Read the model definition and answer for the solid it produces. Units are mm, in the model's axes. Face numbers are marked on the shaded views. A direction names the side the tool comes from. Give positions to 0.01 mm unless a question says otherwise; leave off trailing zeros. Loops run counter-clockwise (first coordinate to the right, second up) from the corner with the lowest first, then second, coordinate; pieces in that order, holes last. Notation, with made-up numbers: (1.5, -1.75) - (25.5, -1.75) arc R16 cw to (25.5, 22.25) - close; hole circle Ø5 at (-32, 64.25). An arc over 180 degrees is marked (long way). Write item = value, one per line. Start each with the question number.
from build123d import *

# Parameters (mm, degrees)
SKETCH_1_R           = 20.68
SKETCH_1_R_2         = 9.68
EXTRUDE_1_DEPTH      = 116.68
SKETCH_11_W          = 27
SKETCH_11_H          = 150
CUT_EXTRUDE_3_DEPTH  = 40
SKETCH_13_W          = 10
SKETCH_13_H          = 128.345013401
CUT_EXTRUDE_7_DEPTH  = 126.614916312
SKETCH_15_W          = 8
SKETCH_15_H          = 68.68
CUT_EXTRUDE_9_DEPTH  = 48
SKETCH_16_W          = 15.549431524
SKETCH_16_H          = 20
SKETCH_16_W_2        = 15.459431524
EXTRUDE_4_DEPTH      = 19.2
SKETCH_17_W          = 19.20851187
SKETCH_17_H          = 14.03
CUT_EXTRUDE_10_DEPTH = 20.2
SKETCH_18_R          = 9.59
CUT_EXTRUDE_11_DEPTH = 121.289430957
SKETCH_21_R          = 2.985
CUT_EXTRUDE_12_DEPTH = 55.2
EXTRUDE_START        = 55.2
SKETCH_24_R          = 20.59
SKETCH_24_R_2        = 9.59
EXTRUDE_2_DEPTH      = 55.2
CUT_EXTRUDE_13_DEPTH = 55.2
SKETCH_26_W          = 10.00851187
SKETCH_26_H          = 41.68
CUT_EXTRUDE_15_DEPTH = 55.2
SKETCH_27_W          = 10
SKETCH_27_H          = 40
CUT_EXTRUDE_16_DEPTH = 55.2
SKETCH_28_W          = 44.880694938
SKETCH_28_H          = 9.608044066
CUT_EXTRUDE_17_DEPTH = 12.2
SKETCH_35_W          = 13.53
SKETCH_35_H          = 20
EXTRUDE_10_DEPTH     = 15
EXTRUDE_11_DEPTH     = 15
SKETCH_37_W          = 9
SKETCH_37_H          = 20
EXTRUDE_12_DEPTH     = 20
SKETCH_38_W          = 9
SKETCH_38_H          = 20
EXTRUDE_13_DEPTH     = 20
SKETCH_42_R          = 2.985
CUT_EXTRUDE_21_DEPTH = 20
CUT_EXTRUDE_23_DEPTH = 138.235841092
SKETCH_45_W          = 3
SKETCH_45_H          = 20
EXTRUDE_14_DEPTH     = 30
SKETCH_46_W          = 3
SKETCH_46_H          = 20
EXTRUDE_15_DEPTH     = 30
SKETCH_47_W          = 33.078221107
SKETCH_47_H          = 20
EXTRUDE_16_DEPTH     = 50
SKETCH_48_W          = 30
SKETCH_48_H          = 20
EXTRUDE_17_DEPTH     = 50
SKETCH_50_W          = 50
SKETCH_50_H          = 20
EXTRUDE_18_DEPTH     = 1
SKETCH_51_W          = 50
SKETCH_51_H          = 20
EXTRUDE_19_DEPTH     = 1
SKETCH_52_W          = 53
SKETCH_52_H          = 14
CUT_EXTRUDE_24_DEPTH = 151.972575738
SKETCH_53_W          = 53
SKETCH_53_H          = 14
CUT_EXTRUDE_25_DEPTH = 151.942387436
SKETCH_54_W          = 40
SKETCH_54_H          = 73.27
CUT_EXTRUDE_26_DEPTH = 147.866192927
SKETCH_56_W          = 13.00851187
SKETCH_56_H          = 20
EXTRUDE_21_DEPTH     = 3.08
SKETCH_58_W          = 44.672014854
SKETCH_58_H          = 95.939897673
CUT_EXTRUDE_28_DEPTH = 149.701311438
SKETCH_59_R          = 9.7
CUT_EXTRUDE_29_DEPTH = 60.553551814
SKETCH_60_W          = 6.504255935
SKETCH_60_H          = 76.35
CUT_EXTRUDE_30_DEPTH = 60.553551814
CUT_EXTRUDE_32_DEPTH = 20
SKETCH_64_W          = 16.20851187
SKETCH_64_H          = 0.09
EXTRUDE_22_DEPTH     = 20
SKETCH_65_W          = 3.495744065
SKETCH_65_H          = 3.26
CUT_EXTRUDE_33_DEPTH = 58.582567932
SKETCH_66_W          = 3.495744065
SKETCH_66_H          = 1.776778893
SKETCH_66_W_2        = 3.503635083
SKETCH_66_H_2        = 1.775
EXTRUDE_23_DEPTH     = 20.2
SKETCH_68_W          = 6.504255935
SKETCH_68_H          = 3.66
CUT_EXTRUDE_34_DEPTH = 20
SKETCH_69_R          = 2.985
CUT_EXTRUDE_35_DEPTH = 124.351086443
SKETCH_70_R          = 2.985
CUT_EXTRUDE_36_DEPTH = 131.530092773


with BuildPart() as part:
    # 草圖1 → 伸長-薄件1 (new body)
    with BuildSketch(Plane(origin=(0, 0, 0), x_dir=(1, 0, 0), z_dir=(0, 1, 0))):
        Circle(SKETCH_1_R)
        Circle(SKETCH_1_R_2, mode=Mode.SUBTRACT)
    extrude(amount=EXTRUDE_1_DEPTH)

    # 草圖11 → 除料-伸長3 (cut)
    with BuildSketch(Plane(origin=(0, 116.68, 0), x_dir=(1, 0, 0), z_dir=(0, 1, 0))):
        with Locations((21.70851187, -44.235815192)):
            Rectangle(SKETCH_11_W, SKETCH_11_H)
    extrude(amount=-CUT_EXTRUDE_3_DEPTH, mode=Mode.SUBTRACT)

    # 草圖13 → 除料-伸長7 (cut, through all)
    with BuildSketch(Plane.XY.offset(21)):
        with Locations((-16, 58.612182466)):
            Rectangle(SKETCH_13_W, SKETCH_13_H)
    extrude(amount=-CUT_EXTRUDE_7_DEPTH, mode=Mode.SUBTRACT)

    # 草圖15 → 除料-伸長9 (cut)
    with BuildSketch(Plane.XY.offset(21)):
        with Locations((-1.395744065, 52.34)):
            Rectangle(SKETCH_15_W, SKETCH_15_H)
    extrude(amount=-CUT_EXTRUDE_9_DEPTH, mode=Mode.SUBTRACT)

    # 草圖16 → 填料-伸長4 (add)
    with BuildSketch(Plane(origin=(8.20851187, 0, 0), x_dir=(0, 0, -1), z_dir=(1, 0, 0))):
        with Locations((12.905284238, 106.68)):
            Rectangle(SKETCH_16_W, SKETCH_16_H)
        with Locations((-12.860284238, 106.68)):
            Rectangle(SKETCH_16_W_2, SKETCH_16_H)
    extrude(amount=-EXTRUDE_4_DEPTH)

    # 草圖17 → 除料-伸長10 (cut)
    with BuildSketch(Plane(origin=(0, 116.68, 0), x_dir=(1, 0, 0), z_dir=(0, 1, 0))):
        with Locations((-1.395744065, -0.045)):
            Rectangle(SKETCH_17_W, SKETCH_17_H)
    extrude(amount=-CUT_EXTRUDE_10_DEPTH, mode=Mode.SUBTRACT)

    # 草圖18 → 除料-伸長11 (cut, through all)
    with BuildSketch(Plane.XZ):
        with Locations(Location((0, 0, 0), (0, 0, 90))):
            Circle(SKETCH_18_R)
    extrude(amount=-CUT_EXTRUDE_11_DEPTH, mode=Mode.SUBTRACT)

    # 草圖21 → 除料-伸長12 (cut)
    with BuildSketch(Plane(origin=(0, 0, -20.68), x_dir=(-1, 0, 0), z_dir=(0, 0, -1))):
        with Locations((1.39148813, 108.73)):
            Circle(SKETCH_21_R)
    extrude(amount=-CUT_EXTRUDE_12_DEPTH, mode=Mode.SUBTRACT)

    # 草圖24 → 伸長-薄件2 (add)
    with BuildSketch(Plane.XZ.offset(EXTRUDE_START)):
        Circle(SKETCH_24_R)
        Circle(SKETCH_24_R_2, mode=Mode.SUBTRACT)
    extrude(amount=-EXTRUDE_2_DEPTH)

    # 草圖25 → 除料-伸長13 (cut)
    with BuildSketch(Plane.XY.offset(21)):
        Polygon((-1.39148813, -11.785), (22.612379708, -11.785), (22.612379708, -63.873337429), (-22.749525245, -63.873337429), (-22.749525245, -11.785), align=None)
    extrude(amount=-CUT_EXTRUDE_13_DEPTH, mode=Mode.SUBTRACT)

    # 草圖26 → 除料-伸長15 (cut)
    with BuildSketch(Plane(origin=(0, 0, 0), x_dir=(1, 0, 0), z_dir=(0, 1, 0))):
        with Locations((-15.995744065, -0.16)):
            Rectangle(SKETCH_26_W, SKETCH_26_H)
    extrude(amount=-CUT_EXTRUDE_15_DEPTH, mode=Mode.SUBTRACT)

    # 草圖27 → 除料-伸長16 (cut)
    with BuildSketch(Plane(origin=(21, 0, 0), x_dir=(0, 0, -1), z_dir=(1, 0, 0))):
        with Locations((0, 41.68)):
            Rectangle(SKETCH_27_W, SKETCH_27_H)
    extrude(amount=-CUT_EXTRUDE_16_DEPTH, mode=Mode.SUBTRACT)

    # 草圖28 → 除料-伸長17 (cut)
    with BuildSketch(Plane(origin=(21, 0, 0), x_dir=(0, 0, -1), z_dir=(1, 0, 0))):
        Rectangle(SKETCH_28_W, SKETCH_28_H)
    extrude(amount=-CUT_EXTRUDE_17_DEPTH, mode=Mode.SUBTRACT)

    # 草圖35 → 填料-伸長10 (add)
    with BuildSketch(Plane.ZY.offset(10.99148813)):
        with Locations((13.825, 106.68)):
            Rectangle(SKETCH_35_W, SKETCH_35_H)
    extrude(amount=EXTRUDE_10_DEPTH)

    # 草圖36 → 填料-伸長11 (add)
    with BuildSketch(Plane.ZY.offset(10.99148813)):
        Polygon((-20.68, 116.68), (-6.97, 116.68), (-6.97, 96.48), (-20.68, 96.68), align=None)
    extrude(amount=EXTRUDE_11_DEPTH)

    # 草圖37 → 填料-伸長12 (add)
    with BuildSketch(Plane.XY.offset(20.59)):
        with Locations((-21.49148813, 106.68)):
            Rectangle(SKETCH_37_W, SKETCH_37_H)
    extrude(amount=EXTRUDE_12_DEPTH)

    # 草圖38 → 填料-伸長13 (add)
    with BuildSketch(Plane(origin=(0, 0, -20.68), x_dir=(-1, 0, 0), z_dir=(0, 0, -1))):
        with Locations((21.49148813, 106.68)):
            Rectangle(SKETCH_38_W, SKETCH_38_H)
    extrude(amount=EXTRUDE_13_DEPTH)

    # 草圖42 → 除料-伸長21 (cut)
    with BuildSketch(Plane(origin=(-16.99148813, 0, 0), x_dir=(0, 0, -1), z_dir=(1, 0, 0))):
        with Locations((30.68, 106.554418142)):
            Circle(SKETCH_42_R)
        with Locations((-30.395640125, 106.68)):
            Circle(SKETCH_42_R)
    extrude(amount=-CUT_EXTRUDE_21_DEPTH, mode=Mode.SUBTRACT)

    # 草圖43 → 除料-伸長23 (cut, through all)
    with BuildSketch(Plane(origin=(0, 116.68, 0), x_dir=(1, 0, 0), z_dir=(0, 1, 0))):
        Polygon((-11, 6.97), (-10.99148813, 20.68), (-10.99148813, 48.096794253), (-28.274756234, 48.096794253), (-28.274756234, -43.270506289), (-11, -43.270506289), align=None)
    extrude(amount=-CUT_EXTRUDE_23_DEPTH, mode=Mode.SUBTRACT)

    # 草圖45 → 填料-伸長14 (add)
    with BuildSketch(Plane.XY.offset(20.59)):
        with Locations((-9.5, 106.68)):
            Rectangle(SKETCH_45_W, SKETCH_45_H)
    extrude(amount=EXTRUDE_14_DEPTH)

    # 草圖46 → 填料-伸長15 (add)
    with BuildSketch(Plane(origin=(0, 0, -20.68), x_dir=(-1, 0, 0), z_dir=(0, 0, -1))):
        with Locations((9.49148813, 106.68)):
            Rectangle(SKETCH_46_W, SKETCH_46_H)
    extrude(amount=EXTRUDE_15_DEPTH)

    # 草圖47 → 填料-伸長16 (add)
    with BuildSketch(Plane.ZY.offset(11)):
        with Locations((34.050889447, 106.68)):
            Rectangle(SKETCH_47_W, SKETCH_47_H)
    extrude(amount=EXTRUDE_16_DEPTH)

    # 草圖48 → 填料-伸長17 (add)
    with BuildSketch(Plane.ZY.offset(10.99148813)):
        with Locations((-35.68, 106.68)):
            Rectangle(SKETCH_48_W, SKETCH_48_H)
    extrude(amount=EXTRUDE_17_DEPTH)

    # 草圖50 → 填料-伸長18 (add)
    with BuildSketch(Plane(origin=(0, 0, 17.511778893), x_dir=(-1, 0, 0), z_dir=(0, 0, -1))):
        with Locations((36, 106.68)):
            Rectangle(SKETCH_50_W, SKETCH_50_H)
    extrude(amount=EXTRUDE_18_DEPTH)

    # 草圖51 → 填料-伸長19 (add)
    with BuildSketch(Plane.XY.offset(-20.68)):
        with Locations((-35.99148813, 106.68)):
            Rectangle(SKETCH_51_W, SKETCH_51_H)
    extrude(amount=EXTRUDE_19_DEPTH)

    # 草圖52 → 除料-伸長24 (cut, through all)
    with BuildSketch(Plane(origin=(0, 116.68, 0), x_dir=(1, 0, 0), z_dir=(0, 1, 0))):
        with Locations((-34.49148813, 43.68)):
            Rectangle(SKETCH_52_W, SKETCH_52_H)
    extrude(amount=-CUT_EXTRUDE_24_DEPTH, mode=Mode.SUBTRACT)

    # 草圖53 → 除料-伸長25 (cut, through all)
    with BuildSketch(Plane(origin=(0, 116.68, 0), x_dir=(1, 0, 0), z_dir=(0, 1, 0))):
        with Locations((-34.5, -43.59)):
            Rectangle(SKETCH_53_W, SKETCH_53_H)
    extrude(amount=-CUT_EXTRUDE_25_DEPTH, mode=Mode.SUBTRACT)

    # 草圖54 → 除料-伸長26 (cut, through all)
    with BuildSketch(Plane(origin=(0, 116.68, 0), x_dir=(1, 0, 0), z_dir=(0, 1, 0))):
        with Locations((-41, 0.045)):
            Rectangle(SKETCH_54_W, SKETCH_54_H)
    extrude(amount=-CUT_EXTRUDE_26_DEPTH, mode=Mode.SUBTRACT)

    # 草圖56 → 填料-伸長21 (add)
    with BuildSketch(Plane(origin=(0, 0, -36.68), x_dir=(-1, 0, 0), z_dir=(0, 0, -1))):
        with Locations((14.495744065, 106.68)):
            Rectangle(SKETCH_56_W, SKETCH_56_H)
    extrude(amount=EXTRUDE_21_DEPTH)

    # 草圖58 → 除料-伸長28 (cut, through all)
    with BuildSketch(Plane.XY.offset(50)):
        with Locations((-0.234953045, 29.661774302)):
            Rectangle(SKETCH_58_W, SKETCH_58_H)
    extrude(amount=-CUT_EXTRUDE_28_DEPTH, mode=Mode.SUBTRACT)

    # 草圖59 → 除料-伸長29 (cut, through all)
    with BuildSketch(Plane.XZ.offset(-77.631723139)):
        Circle(SKETCH_59_R)
    extrude(amount=-CUT_EXTRUDE_29_DEPTH, mode=Mode.SUBTRACT)

    # 草圖60 → 除料-伸長30 (cut, through all)
    with BuildSketch(Plane(origin=(0, 116.68, 0), x_dir=(1, 0, 0), z_dir=(0, 1, 0))):
        with Locations((-17.747872032, 1.585)):
            Rectangle(SKETCH_60_W, SKETCH_60_H)
    extrude(amount=-CUT_EXTRUDE_30_DEPTH, mode=Mode.SUBTRACT)

    # 草圖61 → 除料-伸長32 (cut)
    with BuildSketch(Plane(origin=(0, 116.68, 0), x_dir=(1, 0, 0), z_dir=(0, 1, 0))):
        Polygon((1.92725193, -20.59), (1.92725193, -22.399121663), (-2.174190472, -21.421542421), (-2.174190472, -20.59), align=None)
    extrude(amount=-CUT_EXTRUDE_32_DEPTH, mode=Mode.SUBTRACT)

    # 草圖64 → 填料-伸長22 (add)
    with BuildSketch(Plane(origin=(0, 116.68, 0), x_dir=(1, 0, 0), z_dir=(0, 1, 0))):
        with Locations((0.104255935, -20.635)):
            Rectangle(SKETCH_64_W, SKETCH_64_H)
    extrude(amount=-EXTRUDE_22_DEPTH)

    # 草圖65 → 除料-伸長33 (cut, through all)
    with BuildSketch(Plane(origin=(0, 116.68, 0), x_dir=(1, 0, 0), z_dir=(0, 1, 0))):
        with Locations((-12.747872033, -18.141778893)):
            Rectangle(SKETCH_65_W, SKETCH_65_H)
    extrude(amount=-CUT_EXTRUDE_33_DEPTH, mode=Mode.SUBTRACT)

    # 草圖66 → 填料-伸長23 (add)
    with BuildSketch(Plane(origin=(0, 96.48, 0), x_dir=(1, 0, 0), z_dir=(0, 1, 0))):
        with Locations((-12.747872033, -18.883389447)):
            Rectangle(SKETCH_66_W, SKETCH_66_H)
        with Locations((-12.743926524, 18.7925)):
            Rectangle(SKETCH_66_W_2, SKETCH_66_H_2)
    extrude(amount=EXTRUDE_23_DEPTH)

    # 草圖68 → 除料-伸長34 (cut)
    with BuildSketch(Plane(origin=(0, 116.68, 0), x_dir=(1, 0, 0), z_dir=(0, 1, 0))):
        with Locations((-11.243616098, 37.93)):
            Rectangle(SKETCH_68_W, SKETCH_68_H)
    extrude(amount=-CUT_EXTRUDE_34_DEPTH, mode=Mode.SUBTRACT)

    # 草圖69 → 除料-伸長35 (cut, through all)
    with BuildSketch(Plane(origin=(-7.99148813, 0, 0), x_dir=(0, 0, -1), z_dir=(1, 0, 0))):
        with Locations((28.39, 106.68)):
            Circle(SKETCH_69_R)
        with Locations((-28.635, 106.68)):
            Circle(SKETCH_69_R)
    extrude(amount=-CUT_EXTRUDE_35_DEPTH, mode=Mode.SUBTRACT)

    # 草圖70 → 除料-伸長36 (cut, through all)
    with BuildSketch(Plane(origin=(0, 0, 20.59), x_dir=(-1, 0, 0), z_dir=(0, 0, -1))):
        with Locations((1.39148813, 108.73)):
            Circle(SKETCH_70_R)
    extrude(amount=-CUT_EXTRUDE_36_DEPTH, mode=Mode.SUBTRACT)


solid = part.part
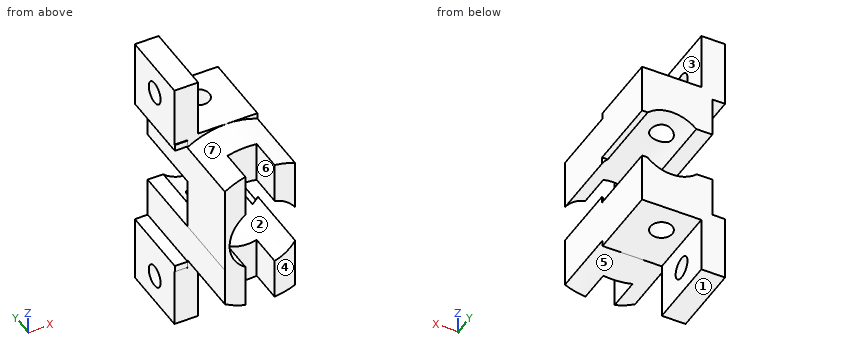
1. A cutting plane is placed at D-D on y = 95.5. Give the vertices of the cut face in (x, z), and give its area (3 significant figures).
2. A tool of negligible diameter and unlimited length cuts with its end or side. For the marked faces 4, 5, 6 and 7, from which of +Z, -Z, +X, -X, +Y, -Y can it reach the whole face along a straight path? Write none if from no direction.
3. A cutting plane is placed at A-A on z = -28.39. Give the vertices of the cut face in (x, y) (3 decimals), and give its area (3 significant figures).
4. A cutting plane is placed at C-C on x = -2.75. Give the vertices of the cut face in (y, z), and give its area (3 significant figures).
5. A cutting plane is placed at B-B on y = 102.5. Give the vertices of the cut face in (x, z) (3 decimals).
6. Consider line 1 along Y through (x, z) = (-1.5, -13.5); line 2 along Z through (x, y) = (-0.5, 91.5); line 3 along X through (y, z) = (86, -15). Determine where each line is inside the solid, lowest interval first. Write a range as [from, to].
7. For a pull along X with two mould halves and no side action, classify the marked faces 1, 2 and 3 as released by +X, released by -X, zero draft, split by the parting line, or undercut.
8. Given P1, Ø7, axis at x = -8, z = -24, coming from the -Y side; P2, Ø1, axis at x = -5, y = 104, coming from the +Z side; P3, Ø17, axis at y = 106.5, z = -30.5, coming from the +X side; P4, Ø8, axis at y = 112, z = -22.5, coming from the +X side, each flat-ended and moving along its own axis, determine where each tip first touches the part or whether it passes through.
Reply:
q1.outline = (-11, -6.97) - (-10.99, -17.52) arc R20.68 ccw to (8.21, -18.98) - (8.21, -5.17) arc R9.7 cw (long way) to (8.21, 5.17) - (8.21, 18.98) arc R20.68 ccw to (-11, 17.51) - close
q1.area = 478 mm^2
q2.face_4 = +Z, -Z, +X, -X, -Y
q2.face_5 = -Z, -Y
q2.face_6 = +Z, -Z, -Y
q2.face_7 = +Z, -Y
q3.outline = (-14.496, 96.68) - (-7.991, 96.68) - (-7.991, 103.695) - (-14.496, 103.695) - close; (-14.496, 109.665) - (-7.991, 109.665) - (-7.991, 116.68) - (-14.496, 116.68) - close
q3.area = 91.3 mm^2
q4.outline = (86.68, -20.5) - (96.68, -20.5) - (96.68, -20.68) - (106.07, -20.68) - (106.07, -9.3) - (86.68, -9.3) - close; (86.68, 9.3) - (106.07, 9.3) - (106.07, 20.68) - (96.68, 20.68) - (96.68, 20.5) - (86.68, 20.5) - close; (111.39, -20.68) - (116.68, -20.68) - (116.68, -9.3) - (111.39, -9.3) - close; (111.39, 9.3) - (116.68, 9.3) - (116.68, 20.68) - (111.39, 20.68) - close
q4.area = 558 mm^2
q5.outline = (-14.496, -36.1) - (-7.991, -36.1) - (-7.991, -20.68) - (8.209, -20.68) - (8.209, -6.97) - (6.746, -6.97) arc R9.7 cw to (-6.746, -6.97) - (-11, -6.97) - (-10.993, -17.905) - (-14.496, -17.905) - close; (-14.496, 17.995) - (-11, 17.995) - (-11, 7.06) - (-6.652, 7.06) arc R9.7 cw to (6.652, 7.06) - (8.209, 7.06) - (8.209, 20.68) - (-8, 20.68) - (-8, 36.59) - (-14.496, 36.59) - close
q6.line_1 = [86.68, 105.75], [111.71, 116.68]
q6.line_2 = [-20.67, -9.69], [9.69, 20.67]
q6.line_3 = [-11, -5.4], [2.6, 8.21]
q7.face_1 = zero draft
q7.face_2 = undercut
q7.face_3 = released by +X
q8.P1 = 96.68
q8.P2 = 20.68
q8.P3 = -7.99
q8.P4 = 8.21
